from build123d import *

# Parameters (mm, degrees)
F1_DEPTH = 38.1
F2_R     = 12.7
F3_R     = 25.4
F4_R     = 17.4625
F5_DEPTH = 721.6628119641
F6_R     = 12.7
F7_DEPTH = 224.2374025718


with BuildPart() as f1:
    # F0 (on Front) → F1 (new body, symmetric)
    with BuildSketch(Plane.XZ):
        Polygon((-298.3877922661, 118.1658460197), (-45.6175838582, 205.2016085916), (132.4110161418, 205.2016085916), (385.1740196981, 118.1683268491), (385.1740196981, 0.0176868491), (404.2240196981, 0.0176868491), (404.2240196981, 131.7565597925), (135.5988928448, 224.2516085916), (-48.8054605612, 224.2516085916), (-317.4377922661, 131.7540789632), (-317.4377922661, 0.0152060197), (-298.3877922661, 0.0152060197), align=None)
    extrude(amount=F1_DEPTH, both=True)

    # F2
    f2_edges = [f1.edges().sort_by_distance(p)[0] for p in [
        (-298.387792, 0, 118.165846),
        (-45.617584, 0, 205.201609),
        (132.411016, 0, 205.201609),
        (385.17402, 0, 118.168327),
    ]]
    fillet(f2_edges, radius=F2_R)

    # F3
    f3_edges = [f1.edges().sort_by_distance(p)[0] for p in [
        (-317.437792, 0, 131.754079),
        (-48.805461, 0, 224.251609),
        (135.598893, 0, 224.251609),
        (404.22402, 0, 131.75656),
    ]]
    fillet(f3_edges, radius=F3_R)

    # F4 (on face) → F5 (cut, through all)
    with BuildSketch(Plane.YZ.offset(404.2240196981)):
        with Locations((0, 40.5980758369)):
            Circle(F4_R)
    extrude(amount=-F5_DEPTH, mode=Mode.SUBTRACT)

    # F6 (on face) → F7 (cut, through all)
    with BuildSketch(Plane.XY.offset(224.2516085916)):
        with Locations((39.2650417094, 0)):
            Circle(F6_R)
    extrude(amount=-F7_DEPTH, mode=Mode.SUBTRACT)


solid = f1.part
Build history of the part. All positions in model axes, mm. A direction names the side the tool comes from. Coordinates: 2 decimals unless noted, no trailing zeros. Write each loop counter-clockwise with the first axis right and the second up, starting at its lowest first coordinate (ties: lowest second). Pieces come first, ordered by that corner, then holes.
(1) Cut at D-D on z = 188. List the corners of the cut face in (x, y).
(2) Drill centre lines: line 1 (X direction, y = 15.5, z = 12.5); line 2 (Z direction, x = -310.75, y = 0); line 3 (Z direction, x = 55.5, y = -23). Where is each one in solid material? Low to high.
(3) Pin check, flat tips, straight feed: pin 1 Ø8 at (x, y) = (-207, -6.5) entering from -Z; pin 2 Ø10 at (x, y) = (-130, 18) entering from -Z; pin 3 Ø1.5 at (x, y) = (79, 27.5) entering from -Z. Stop position of each tip, or through.
(4) Mould opens along X. For faces 3 (the flat face through (-170.42, -0.53, 162.23)), 4 (the flat face through (-308, -1, 0.015)), 5 (the cylindrical face through (399.37, -0.53, 128.57)), 6 (the flat face through (-317.438, -9, 58)) say: pulls with the +X half, pulls with the -X half, needs draft (parallel to the pull), parting line crosses it, or undercut.
(5) Cut at B-B on y = 0. State how many separate pieces and enclosed holes the cut face has, and give its area (3 significant figures).
(6) Cut at A-A on z = 90. List the corners of the cut face in (x, y), and give its area (3 significant figures).
(7) 3-axis set-ups, long thin cutter, end or side, ignore diameter. For faces 1 (the cylindrical face through (394.83, -3.79, 23.55)), 2 (the flat face through (-298.388, -1, 66)): which of +Z, -Z, +X, -X, +Y, -Y reach the whole face in a straight line?
(8) Cut at C-C on y = 32. List the corners of the cut face in (x, z), and give its area (3 significant figures).
Working result:
1. outline: (-154.09, -38.1) - (-95.57, -38.1) - (-95.57, 38.1) - (-154.09, 38.1) - close; (182.37, -38.1) - (240.88, -38.1) - (240.88, 38.1) - (182.37, 38.1) - close
2. line 1: x = -317.44 to -298.39, 385.17 to 404.22
2. line 2: z = 0.02 to 23.14, 58.06 to 130.81
2. line 3: z = 205.2 to 224.25
3. pin 1: stops at z = 148.26
3. pin 2: stops at z = 174.42
3. pin 3: stops at z = 205.2
4. face 3: undercut
4. face 4: needs draft
4. face 5: pulls with the +X half
4. face 6: pulls with the -X half
5. separate pieces: 4
5. enclosed holes: 0
5. area: 16,800 mm2
6. outline: (-317.44, -38.1) - (-298.39, -38.1) - (-298.39, 38.1) - (-317.44, 38.1) - close; (385.17, -38.1) - (404.22, -38.1) - (404.22, 38.1) - (385.17, 38.1) - close
6. area: 2,900 mm2
7. face 1: +X, -X
7. face 2: -Z, +Y, -Y
8. outline: (-317.44, 0.02) - (-298.39, 0.02) - (-298.39, 109.11) arc R12.7 cw to (-289.82, 121.12) - (-47.63, 204.51) arc R12.7 cw to (-43.49, 205.2) - (130.29, 205.2) arc R12.7 cw to (134.42, 204.51) - (376.61, 121.12) arc R12.7 cw to (385.17, 109.11) - (385.17, 0.02) - (404.22, 0.02) - (404.22, 113.64) arc R25.4 ccw to (387.09, 137.66) - (139.62, 222.87) arc R25.4 ccw to (131.35, 224.25) - (-44.55, 224.25) arc R25.4 ccw to (-52.82, 222.87) - (-300.31, 137.65) arc R25.4 ccw to (-317.44, 113.64) - close
8. area: 18,600 mm2
